from build123d import *

# Parameters (mm, degrees)
SKETCH1_W           = 200
SKETCH1_H           = 100
BOSS_EXTRUDE1_DEPTH = 5
SKETCH2_R           = 2.5
CUT_EXTRUDE1_DEPTH  = 112.915146428
SKETCH3_R           = 3.75
CUT_EXTRUDE2_DEPTH  = 4
FILLET1_R           = 3


with BuildPart() as part:
    # Sketch1 → Boss-Extrude1 (new body)
    with BuildSketch(Plane(origin=(0, 0, 0), x_dir=(1, 0, 0), z_dir=(0, 1, 0))):
        Rectangle(SKETCH1_W, SKETCH1_H)
    extrude(amount=BOSS_EXTRUDE1_DEPTH)

    # Sketch2 → Cut-Extrude1 (cut, through all)
    with BuildSketch(Plane(origin=(0, 5, 0), x_dir=(1, 0, 0), z_dir=(0, 1, 0))):
        with Locations(Location((-93, 43, 0), (0, 0, 270))):
            Circle(SKETCH2_R)
        with Locations(Location((-45, -35, 0), (0, 0, 270))):
            Circle(SKETCH2_R)
        with Locations(Location((93, 43, 0), (0, 0, 90))):
            Circle(SKETCH2_R)
        with Locations(Location((45, -35, 0), (0, 0, 90))):
            Circle(SKETCH2_R)
    extrude(amount=-CUT_EXTRUDE1_DEPTH, mode=Mode.SUBTRACT)

    # Sketch3 → Cut-Extrude2 (cut)
    with BuildSketch(Plane(origin=(0, 5, 0), x_dir=(1, 0, 0), z_dir=(0, 1, 0))):
        with Locations(Location((-93, 43, 0), (0, 0, 270))):
            Circle(SKETCH3_R)
        with Locations(Location((-45, -35, 0), (0, 0, 270))):
            Circle(SKETCH3_R)
        with Locations(Location((45, -35, 0), (0, 0, 90))):
            Circle(SKETCH3_R)
        with Locations(Location((93, 43, 0), (0, 0, 90))):
            Circle(SKETCH3_R)
    extrude(amount=-CUT_EXTRUDE2_DEPTH, mode=Mode.SUBTRACT)

    # Fillet1
    fillet1_edges = [part.edges().sort_by_distance(p)[0] for p in [
        (0, 5, 50),
        (0, 5, -50),
    ]]
    fillet(fillet1_edges, radius=FILLET1_R)


solid = part.part
The listing builds one solid part. Answer for the finished solid, in the listing's coordinates (mm). A direction names the side the tool comes from. Give positions to 0.01 mm unless a question says otherwise; leave off trailing zeros. Loops run counter-clockwise (first coordinate to the right, second up) from the corner with the lowest first, then second, coordinate; pieces in that order, holes last.
Item 1: A cutting plane is placed at B-B (x = -93). Give the vertices of the cut face in (y, z).
Derived:
outline: (0, -50) - (2, -50) arc R3 ccw to (5, -47) - (5, -46.75) - (1, -46.75) - (1, -45.5) - (0, -45.5) - close; (0, -40.5) - (1, -40.5) - (1, -39.25) - (5, -39.25) - (5, 47) arc R3 ccw to (2, 50) - (0, 50) - close
Item 2: A cutting plane is placed at A-A (z = 35). Give the vertices of the cut face in (x, y).
Derived:
outline: (-100, 0) - (-47.5, 0) - (-47.5, 1) - (-48.75, 1) - (-48.75, 5) - (-100, 5) - close; (-42.5, 0) - (42.5, 0) - (42.5, 1) - (41.25, 1) - (41.25, 5) - (-41.25, 5) - (-41.25, 1) - (-42.5, 1) - close; (47.5, 0) - (100, 0) - (100, 5) - (48.75, 5) - (48.75, 1) - (47.5, 1) - close
Item 3: Find the intervals of material crossed by line 1 along X through (y, z) = (0.85, -43); line 2 along X through (y, z) = (2.45, 35); line 3 along Z through (x, y) = (45, 4.1), in increasing order.
Derived:
line 1: x = -100 to -95.5, -90.5 to 90.5, 95.5 to 100
line 2: x = -100 to -48.75, -41.25 to 41.25, 48.75 to 100
line 3: z = -49.14 to 31.25, 38.75 to 49.14
Item 4: Each of these flat-tipped pins is pushed along its axis until it touches: pin 1 Ø4 at (x, z) = (-93.5, -44) entering from +Y; pin 2 Ø1 at (x, y) = (-31, 3.5) entering from -Z. Where does it stop, or does it pass through?
Derived:
pin 1: stops at y = 1
pin 2: stops at z = -49.83
Item 5: A tool of negligible diameter and unlimited length cuts with its end or side. For faces 1 (the flat face through (-100, 2, 1)), 2 (the flat face through (45, 1, 38)), from which of +Z, -Z, +X, -X, +Y, -Y can it reach the whole face along a straight path? Write none if from no direction.
Derived:
face 1: +Z, -Z, -X, +Y, -Y
face 2: +Y
Item 6: A cutting plane is placed at C-C (y = 3.9). Give the vertices of the cut face in (x, z).
Derived:
outline: (-100, -49.32) - (100, -49.32) - (100, 49.32) - (-100, 49.32) - close; hole circle Ø7.5 at (-93, -43); hole circle Ø7.5 at (-45, 35); hole circle Ø7.5 at (45, 35); hole circle Ø7.5 at (93, -43)
